For this review, take the finished solid that the model builds, in its own axes (mm). A direction names the side the tool comes from. Round coordinates to 2 decimals unless told otherwise and drop trailing zeros. Order: outer loops, then holes, each group sorted by start corner. A loop starts at its lowest first (then second) coordinate and runs counter-clockwise, first axis right, second up. Notation, with made-up numbers: M -38,-32 L 12,-32 A30 cw 12,-9 Z; hole C 83,82 d7. An arc over 180 degrees is marked long. Put each result on its own line as item: value.
Autodesk Inventor part; units mm, degrees
ref_plane "YZ Plane" through (0, 0, 0) normal (1, 0, 0) x (0, 1, 0)
ref_plane "XZ Plane" through (0, 0, 0) normal (0, 1, 0) x (-1, 0, 0)
ref_plane "XY Plane" through (0, 0, 0) normal (0, 0, 1) x (1, 0, 0)
sketch "Sketch1" plane through (0, 0, 0) normal (0, 0, 1) x (1, 0, 0)
  circle A0 centre (0, 0) radius 25
  circle A1 centre (150, 0) radius 15
  line L0 (0, 0) -> (150, 0)
  line L1 (0.7508, 24.9887) -> (150.9983, 14.9667)
  line L2 (0.7508, -24.9887) -> (150.9983, -14.9667)
  point P0 (0.7508, -24.9887)
  point P1 (150.9983, -14.9667)
  point P2 (2.5747, -24.8671)
  point P3 (2.5747, 24.8671)
  dimension "d10" = 15
  dimension "d11" = 25
  dimension "d9" = 150
extrude "Extrusion1" add sketch "Sketch1" along normal blind 6
sketch "Sketch2" plane through (0, 0, 6) normal (0, 0, 1) x (1, 0, 0)
  circle A0 centre (0, 0) radius 1.75
  arc A1 (150.9983, -14.9667) -> (150.9983, 14.9667) centre (150, 0) ccw
  circle A2 centre (150, 0) radius 1.75
  point P0 (293.3543, -13.4475)
  point P1 (293.3543, 13.4475)
  point P2 (250.3596, -14.9957)
  point P3 (250.3596, 14.9957)
  dimension "d5" = 3.5
  dimension "d6" = 3.5
extrude "Extrusion2" cut sketch "Sketch2" against normal blind 6
sketch "Sketch4" plane through (0, 0, 6) normal (0, 0, 1) x (1, 0, 0)
  circle A0 centre (0, 0) radius 12.5
  circle A1 centre (0, 0) radius 1.75
  circle A2 centre (0, 0) radius 30
  circle A3 centre (150, 0) radius 1.75
  circle A4 centre (150, 0) radius 9.913
  arc A5 (150.9983, -14.9667) -> (150.9983, 14.9667) centre (150, 0) ccw
  circle A6 centre (150, 0) radius 22.5
  line L0 (150.9983, 14.9667) -> (2.5747, 24.8671)
  line L1 (18.2342, 23.8225) -> (134.265, 16.0829)
  line L2 (18.2342, -23.8225) -> (134.265, -16.0829)
  line L3 (2.5747, -24.8671) -> (150.9983, -14.9667)
  dimension "d20" = 25
  dimension "d21" = 60
  dimension "d22" = 19.826
  dimension "d23" = 45
extrude "Extrusion4" add sketch "Sketch4" along normal blind 48.5 contours A2 L0 A6 L2
properties part number "Tibia"
(1) Add section D-D on x = 25.5. Give the boundary of the cut face in (y, z).
A:
outline: M -23.34,0 L 23.34,0 L 23.34,54.5 L 15.8,54.5 L 15.8,6 L -15.8,6 L -15.8,54.5 L -23.34,54.5 Z
(2) To check wall thickness, follow L1, parallel to Z at x = 10, y = -13; L2, parallel to Y at x = 150, z = 4.5; L3, parallel to X at y = -11.5, z = 21.5. State the ranges of each line that lie inside material, in increasing order.
A:
L1: z = 0 to 6
L2: y = -15.03 to -1.75, 1.75 to 15.03
L3: x = 27.71 to 130.66
(3) Insertion check: pin 1 Ø5 at (x, z) = (30, 12.5) entering from +Y; pin 2 Ø5 at (y, z) = (4, 16.5) entering from -X; pin 3 Ø8 at (y, z) = (19.5, 40.5) entering from -X; pin 4 Ø2 at (x, y) = (150, 0) entering from -Z. Each pin has a flat end and moves straight along its axis. Give the tip position at first contact, or say it passes through.
A:
pin 1: stops at y = 23.2
pin 2: stops at x = 29.29
pin 3: stops at x = 18.65
pin 4: passes through
(4) Add section B-B on y = 0. Give the boundary of the cut face in (x, z), then the cut area to 3 significant figures.
A:
outline: M -25,0 L -1.75,0 L -1.75,6 L -25,6 Z; M 1.75,0 L 148.25,0 L 148.25,6 L 127.5,6 L 127.5,54.5 L 30,54.5 L 30,6 L 1.75,6 Z; M 151.75,0 L 165,0 L 165,6 L 151.75,6 Z
area: 5,830 mm2
(5) Draft analysis for pull direction X (two halves, no side actions). For faces 4 (the face through (165, 0, 3)), 5 (the face through (151.669, 0.526, 3.042)), 6 (the face through (30, 0, 30)), state which applies: released by +X, released by -X, zero draft, split by the parting line, or undercut.
A:
face 4: released by +X
face 5: undercut
face 6: released by -X
(6) For faces 1 (the face through (75, 0, 54.5)), 2 (the face through (127.5, -0.3, 29.9)), 3 (the face through (2, 0, 6)), list the 3-axis set-ups (+Z, -Z, +X, -X, +Y, -Y) from which the entire face can be reached by the end or side of a thin tool; tool diameter is ignored.
A:
face 1: +Z, +X, -X, +Y, -Y
face 2: +Z, +X
face 3: +Z, -X
(7) Add section C-C on y = 22. Give the boundary of the cut face in (x, z).
A:
outline: M -11.87,0 L 45.56,0 L 45.56,54.5 L 20.4,54.5 L 20.4,6 L -11.87,6 Z
(8) Add section A-A on x = 0. Give the boundary of the cut face in (y, z), then the cut area to 3 significant figures.
A:
outline: M -25,0 L -1.75,0 L -1.75,6 L -25,6 Z; M 1.75,0 L 25,0 L 25,6 L 1.75,6 Z
area: 279 mm2
